from build123d import *

# Parameters (mm, degrees)
F0_R     = 304.8
F0_R_2   = 19.4437
F0_R_3   = 152.4
F1_DEPTH = 25.4
F2_R     = 215.9
F2_R_2   = 152.4
F3_DEPTH = 25.4
F4_R     = 177.8
F4_R_2   = 152.4
F5_DEPTH = 25.4


with BuildPart() as f1:
    # F0 (on Front) → F1 (new body, symmetric)
    with BuildSketch(Plane.XZ):
        Circle(F0_R)
        with Locations((-179.605122, -179.605122)):
            Circle(F0_R_2, mode=Mode.SUBTRACT)
        with Locations((0, -254)):
            Circle(F0_R_2, mode=Mode.SUBTRACT)
        with Locations((179.605122, -179.605122)):
            Circle(F0_R_2, mode=Mode.SUBTRACT)
        with Locations((-254, 0)):
            Circle(F0_R_2, mode=Mode.SUBTRACT)
        with Locations((-179.605122, 179.605122)):
            Circle(F0_R_2, mode=Mode.SUBTRACT)
        Circle(F0_R_3, mode=Mode.SUBTRACT)
        with Locations((254, 0)):
            Circle(F0_R_2, mode=Mode.SUBTRACT)
        with Locations((0, 254)):
            Circle(F0_R_2, mode=Mode.SUBTRACT)
        with Locations((179.605122, 179.605122)):
            Circle(F0_R_2, mode=Mode.SUBTRACT)
    extrude(amount=F1_DEPTH, both=True)

    # F2 (on face) → F3 (join)
    with BuildSketch(Plane.XZ.offset(25.4)):
        Circle(F2_R)
        Circle(F2_R_2, mode=Mode.SUBTRACT)
    extrude(amount=F3_DEPTH)

    # F4 (on face) → F5 (join)
    with BuildSketch(Plane(origin=(0, 25.4, 0), x_dir=(-1, 0, 0), z_dir=(0, 1, 0))):
        Circle(F4_R)
        Circle(F4_R_2, mode=Mode.SUBTRACT)
    extrude(amount=F5_DEPTH)


solid = f1.part
Verification items for the finished model (mm, model axes). A direction names the side the tool comes from. Coordinates: 2 decimals unless noted, no trailing zeros. Order: outer loops, then holes, each group sorted by start corner. A loop starts at its lowest first (then second) coordinate and runs counter-clockwise, first axis right, second up. Notation, with made-up numbers: (18.5, 8.5) -> (57.5, 8.5) arc R18 ccw to (57.5, 41.5) -> close; hole circle Ø2 at (-5, 70). An arc over 180 degrees is marked (long way). Put each result on its own line as item: value. Start each with the question number.
1. Cross-section at D-D, the plane x = -254. Record the boundary of the cut face in (y, z), then the cut area to 3 significant figures.
2. Material ranges on L1, parallel to Z at x = 0, y = -19; L2, parallel to Z at x = -168, y = -3; L3, parallel to Y at x = -174, z = 208.5, recorded low to high. Write a range as [from, to].
3. Cross-section at C-C, the plane z = 254. Record the boundary of the cut face in (x, y).
4. Access from +Z, -Z, +X, -X, +Y, -Y to the whole of each face (thin tool, end or side, straight path). Record for faces 4 (the flat face through (-207, -25.4, 72)), 5 (the cylindrical face through (-169.59, 37.92, 53.41)), 6 (the cylindrical face through (-199.03, 0.36, -178.75)).
5. Cross-section at A-A, the plane z = 0. Record the boundary of the cut face in (x, y), then the cut area to 3 significant figures.
6. Cross-section at B-B, the plane x = 0. Record the boundary of the cut face in (y, z), then the cut area to 3 significant figures.
7. Mould release check, pull along Z, two halves, no side actions. Record for faces 1 (the cylindrical face through (234.575, 0.356, 0.855)), 2 (the flat face through (45, -50.8, 147)), 3 (the cylindrical face through (-159.127, -37.922, 145.915)): released by +Z, released by -Z, zero draft, split by the parting line, or undercut.
8. Go/stop test with flat-tipped pins: pin 1 Ø1 at (y, z) = (-2, 180.5) entering from +X; pin 2 Ø2 at (y, z) = (24, 217) entering from +X; pin 3 Ø1.5 at (x, y) = (181, 27.5) entering from -Z; pin 4 Ø4 at (x, z) = (209.5, 181.5) entering from -Y. Record where each tip stops, or that it passes through.
Computed:
1. outline: (-25.4, -168.48) -> (25.4, -168.48) -> (25.4, -19.44) -> (-25.4, -19.44) -> close; (-25.4, 19.44) -> (25.4, 19.44) -> (25.4, 168.48) -> (-25.4, 168.48) -> close
1. area: 15,100 mm2
2. L1: [-304.8, -273.44], [-234.56, -152.4], [152.4, 234.56], [273.44, 304.8]
2. L2: [-254.32, -195.21], [-164, 164], [195.21, 254.32]
2. L3: [-25.4, 25.4]
3. outline: (-168.48, -25.4) -> (-19.44, -25.4) -> (-19.44, 25.4) -> (-168.48, 25.4) -> close; (19.44, -25.4) -> (168.48, -25.4) -> (168.48, 25.4) -> (19.44, 25.4) -> close
4. face 4: -Y
4. face 5: +Y
4. face 6: +Y, -Y
5. outline: (-304.8, -25.4) -> (-273.44, -25.4) -> (-273.44, 25.4) -> (-304.8, 25.4) -> close; (-234.56, -25.4) -> (-215.9, -25.4) -> (-215.9, -50.8) -> (-152.4, -50.8) -> (-152.4, 50.8) -> (-177.8, 50.8) -> (-177.8, 25.4) -> (-234.56, 25.4) -> close; (152.4, -50.8) -> (215.9, -50.8) -> (215.9, -25.4) -> (234.56, -25.4) -> (234.56, 25.4) -> (177.8, 25.4) -> (177.8, 50.8) -> (152.4, 50.8) -> close; (273.44, -25.4) -> (304.8, -25.4) -> (304.8, 25.4) -> (273.44, 25.4) -> close
5. area: 16,000 mm2
6. outline: (-50.8, -215.9) -> (-25.4, -215.9) -> (-25.4, -234.56) -> (25.4, -234.56) -> (25.4, -177.8) -> (50.8, -177.8) -> (50.8, -152.4) -> (-50.8, -152.4) -> close; (-50.8, 152.4) -> (50.8, 152.4) -> (50.8, 177.8) -> (25.4, 177.8) -> (25.4, 234.56) -> (-25.4, 234.56) -> (-25.4, 215.9) -> (-50.8, 215.9) -> close; (-25.4, -304.8) -> (25.4, -304.8) -> (25.4, -273.44) -> (-25.4, -273.44) -> close; (-25.4, 273.44) -> (25.4, 273.44) -> (25.4, 304.8) -> (-25.4, 304.8) -> close
6. area: 16,000 mm2
7. face 1: undercut
7. face 2: zero draft
7. face 3: split by the parting line
8. pin 1: x = 245.97
8. pin 2: x = 215.05
8. pin 3: through
8. pin 4: y = -25.4
